Geometry check sheet. Reference: the model listing, model coordinates, mm. Coordinates: 2 decimals unless noted, no trailing zeros. Loops run counter-clockwise (first coordinate to the right, second up) from the corner with the lowest first, then second, coordinate; pieces in that order, holes last. Notation, with made-up numbers: M -14.75,35.5 L 23.25,35.5 A9 ccw 23.25,51.5 Z; hole C 88.5,15.5 d2. An arc over 180 degrees is marked long. Use CSV: the item, a comma, the result in double quotes.
```python
from build123d import *

# Parameters (mm, degrees)
SKETCH1_R           = 1.6
SKETCH1_R_2         = 1.25
BOSS_EXTRUDE1_DEPTH = 6


with BuildPart() as part:
    # Sketch1 → Boss-Extrude1 (new body)
    with BuildSketch(Plane(origin=(0, 0, 0), x_dir=(1, 0, 0), z_dir=(0, 1, 0))):
        with BuildLine():
            Line((0, 0), (-60, 0))
            ThreePointArc((-60, 0), (-70, 10), (-60, 20))
            Line((-60, 20), (0, 20))
            ThreePointArc((0, 20), (10, 10), (0, 0))
        make_face()
        with Locations((-60, 10)):
            Circle(SKETCH1_R, mode=Mode.SUBTRACT)
        with Locations((-60, 17)):
            Circle(SKETCH1_R_2, mode=Mode.SUBTRACT)
        with Locations((-60, 3)):
            Circle(SKETCH1_R_2, mode=Mode.SUBTRACT)
        with Locations((-67, 10)):
            Circle(SKETCH1_R_2, mode=Mode.SUBTRACT)
        with Locations((-53, 10)):
            Circle(SKETCH1_R_2, mode=Mode.SUBTRACT)
        with Locations((0, 10)):
            Circle(SKETCH1_R, mode=Mode.SUBTRACT)
        with Locations((-30, 10)):
            Circle(SKETCH1_R, mode=Mode.SUBTRACT)
    extrude(amount=BOSS_EXTRUDE1_DEPTH)


solid = part.part
```
1. Section check D-D, the plane z = -3. Record the cut outline in (x, y).
The answers:
outline,"M -67.14,0 L -61.25,0 L -61.25,6 L -67.14,6 Z; M -58.75,0 L 7.14,0 L 7.14,6 L -58.75,6 Z"
2. Section check A-A, the plane x = -30. Record the cut outline in (y, z).
The answers:
outline,"M 0,-20 L 6,-20 L 6,-11.6 L 0,-11.6 Z; M 0,-8.4 L 6,-8.4 L 6,0 L 0,0 Z"
3. Release check for a two-part mould opening along Z. For faces 1 (the flat face through (-29, 0, -8)), 2 (the cylindrical face through (-70, 3, -10)), 3 (the cylindrical face through (-58.81, 2.96, -17.38)), 4 (the cylindrical face through (-51.81, 2.96, -10.38)) record: +Z half, -Z half, draft (parallel to the pull), parting line (faces both ways), or undercut.
The answers:
face 1,"draft"
face 2,"parting line"
face 3,"undercut"
face 4,"undercut"
4. Section check C-C, the plane y = 5. Record the cut outline in (x, z), plus the area to 3 significant figures.
The answers:
outline,"M -60,-20 L 0,-20 A10 ccw 0,0 L -60,0 A10 ccw Z; hole C -67,-10 d2.5; hole C -60,-10 d3.2; hole C -60,-17 d2.5; hole C -60,-3 d2.5; hole C -53,-10 d2.5; hole C -30,-10 d3.2; hole C 0,-10 d3.2"
area,"1,470 mm^2"
5. Gauge pin test, flat end, axial feed: P1, Ø3, axis at x = -60, z = -3, coming from the -Y side. Record the tip position at first contact, or that the pin passes through.
The answers:
P1,"y = 0"
6. Section check B-B, the plane z = -10. Record the cut outline in (x, y), plus the area to 3 significant figures.
The answers:
outline,"M -70,0 L -68.25,0 L -68.25,6 L -70,6 Z; M -65.75,0 L -61.6,0 L -61.6,6 L -65.75,6 Z; M -58.4,0 L -54.25,0 L -54.25,6 L -58.4,6 Z; M -51.75,0 L -31.6,0 L -31.6,6 L -51.75,6 Z; M -28.4,0 L -1.6,0 L -1.6,6 L -28.4,6 Z; M 1.6,0 L 10,0 L 10,6 L 1.6,6 Z"
area,"392 mm^2"
7. Thickness scan on line 1 (Z direction, x = -60, y = 3.1); line 2 (Z direction, x = -30, y = 4.85); line 3 (Z direction, x = -53, y = 2.25). Record the ranges inside material, lowest first. Write a range as [from, to].
The answers:
line 1,"[-20, -18.25], [-15.75, -11.6], [-8.4, -4.25], [-1.75, 0]"
line 2,"[-20, -11.6], [-8.4, 0]"
line 3,"[-20, -11.25], [-8.75, 0]"
